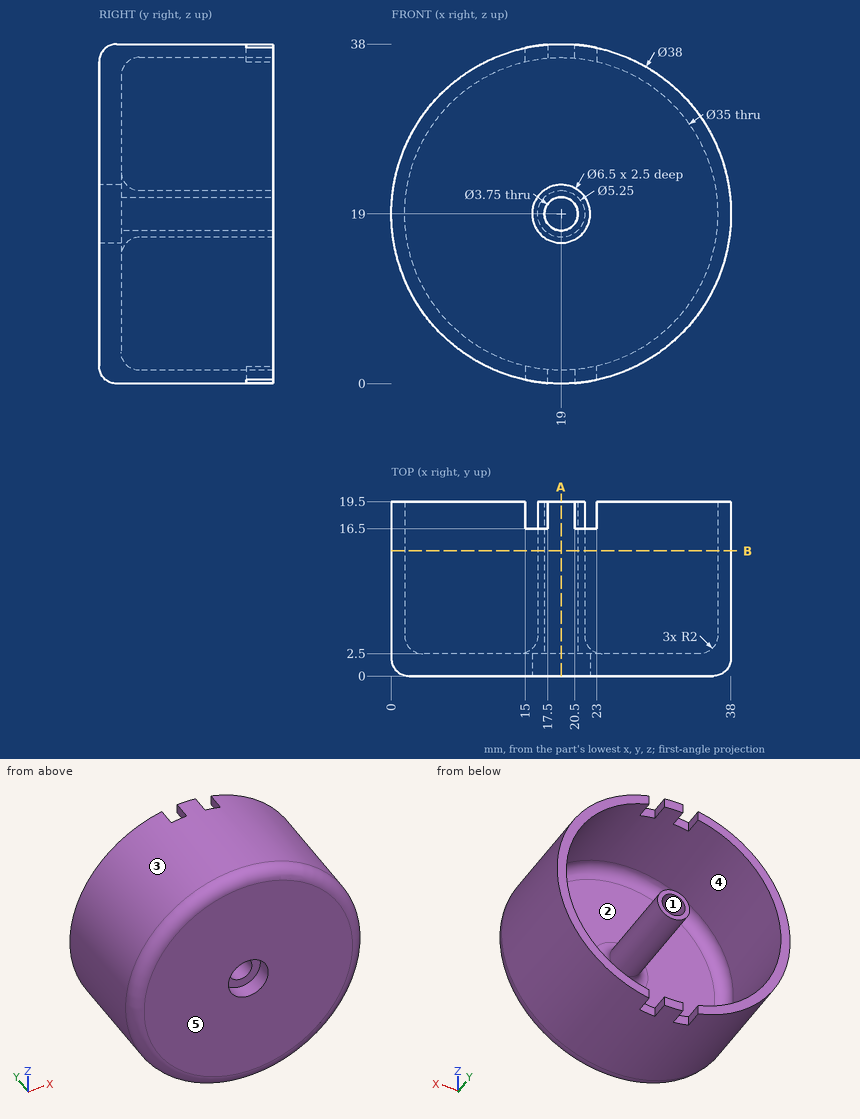
Verification items for this drawing (mm, ordinates from the low corner). A direction names the side the tool comes from. Give positions to 0.01 mm unless a question says otherwise; leave off trailing zeros. Write each loop counter-clockwise with the first axis right and the second up, starting at its lowest first coordinate (ties: lowest second). Pieces come first, ordered by that corner, then holes.
1) Go/stop test with flat-tipped pins: pin 1 Ø10 at (y, z) = (13, 25.5) entering from +X; pin 2 Ø3 at (x, z) = (18, 20) entering from -Y; pin 3 Ø1.7 at (y, z) = (17.5, 37) entering from -X. Record where each tip stops, or that it passes through.
Values follow:
pin 1: stops at x = 37.94
pin 2: stops at y = 2.5
pin 3: stops at x = 10.82
2) Thickness scan on line 1 (X direction, y = 10, z = 19) (3 decimals); line 2 (Y direction, x = 7, z = 9); line 3 (Z direction, x = 35, y = 18.75). Record the ranges inside material, lowest first.
Values follow:
line 1: x = 0 to 1.5, 16.375 to 17.125, 20.875 to 21.625, 36.5 to 38
line 2: y = 0 to 2.5
line 3: z = 8.75 to 11.91, 26.09 to 29.25
3) Release check for a two-part mould opening along X. For the marked faces 3, 4 and 5 record: released by +X, released by -X, zero draft, split by the parting line, or undercut.
Values follow:
face 3: split by the parting line
face 4: undercut
face 5: zero draft
4) Set-up check for the marked faces 1 and 2: record each of +Z, -Z, +X, -X, +Y, -Y from which the full face is reachable in a straight line by a thin tool's end or side.
Values follow:
face 1: +Y, -Y
face 2: +Y
5) Cross-section at B-B (y = 14). Record the boundary of the cut face in (x, z) (3 decimals).
Values follow:
outline: circle Ø38 at (19, 19); circle Ø5.25 at (19, 19); hole circle Ø35 at (19, 19); hole circle Ø3.75 at (19, 19)
6) Cross-section at A-A (x = 19). Record the boundary of the cut face in (y, z) (3 decimals).
Values follow:
outline: (0, 2) arc R2 ccw to (2, 0) - (19.5, 0) - (19.5, 1.5) - (4.5, 1.5) arc R2 cw to (2.5, 3.5) - (2.5, 14.375) arc R2 cw to (4.5, 16.375) - (19.5, 16.375) - (19.5, 17.125) - (2.5, 17.125) - (2.5, 15.75) - (0, 15.75) - close; (0, 22.25) - (2.5, 22.25) - (2.5, 20.875) - (19.5, 20.875) - (19.5, 21.625) - (4.5, 21.625) arc R2 cw to (2.5, 23.625) - (2.5, 34.5) arc R2 cw to (4.5, 36.5) - (19.5, 36.5) - (19.5, 38) - (2, 38) arc R2 ccw to (0, 36) - close
